Job drawing, mm, ordinate dimensions from the low corner. One solid piece. A direction names the side the tool comes from. Give positions to 0.01 mm unless a question says otherwise; leave off trailing zeros. Order: outer loops, then holes, each group sorted by start corner. A loop starts at its lowest first (then second) coordinate and runs counter-clockwise, first axis right, second up. Notation, with made-up numbers: M -37.5,24 L -3.5,24 A24 cw -3.5,47 Z; hole C 68.5,-38 d3. An arc over 180 degrees is marked long. Use CSV: the item, a comma, the result in double quotes. Start each with the question number.
Item 1: Band-saw the part on A-A on x = 38.5. Write the cut outline in (y, z) (3 decimals), plus the area to 3 significant figures.
Item 2: Band-saw the part on D-D on x = 7. Write the cut outline in (y, z) (3 decimals).
Item 3: Band-saw the part on B-B on y = 1.55. Write the cut outline in (x, z), plus the area to 3 significant figures.
Item 4: Which spindle directions (+Z, -Z, +X, -X, +Y, -Y) get a long thin tool onto all of the face, cutting with end or side? Do the marked faces 1, 2, 3 and 4. Say none if no direction does.
Item 5: Wall check: line 1 along Z through (x, y) = (34.5, 2.6); line 2 along X through (y, z) = (2, 51). Give the ranges that are in metal, low to high.
Item 6: Pin check, flat tips, straight feed: P1, Ø1, axis at x = 48.5, y = 2, coming from the -Z side (3 decimals); P2, Ø1, axis at x = 43.5, y = 2, coming from the +Z side (3 decimals); P3, Ø2, axis at y = 4, z = 14.5, coming from the -X side. Stop position of each tip, or through.
Item 7: Band-saw the part on C-C on z = 66.5. Write the cut outline in (x, y) (3 decimals).
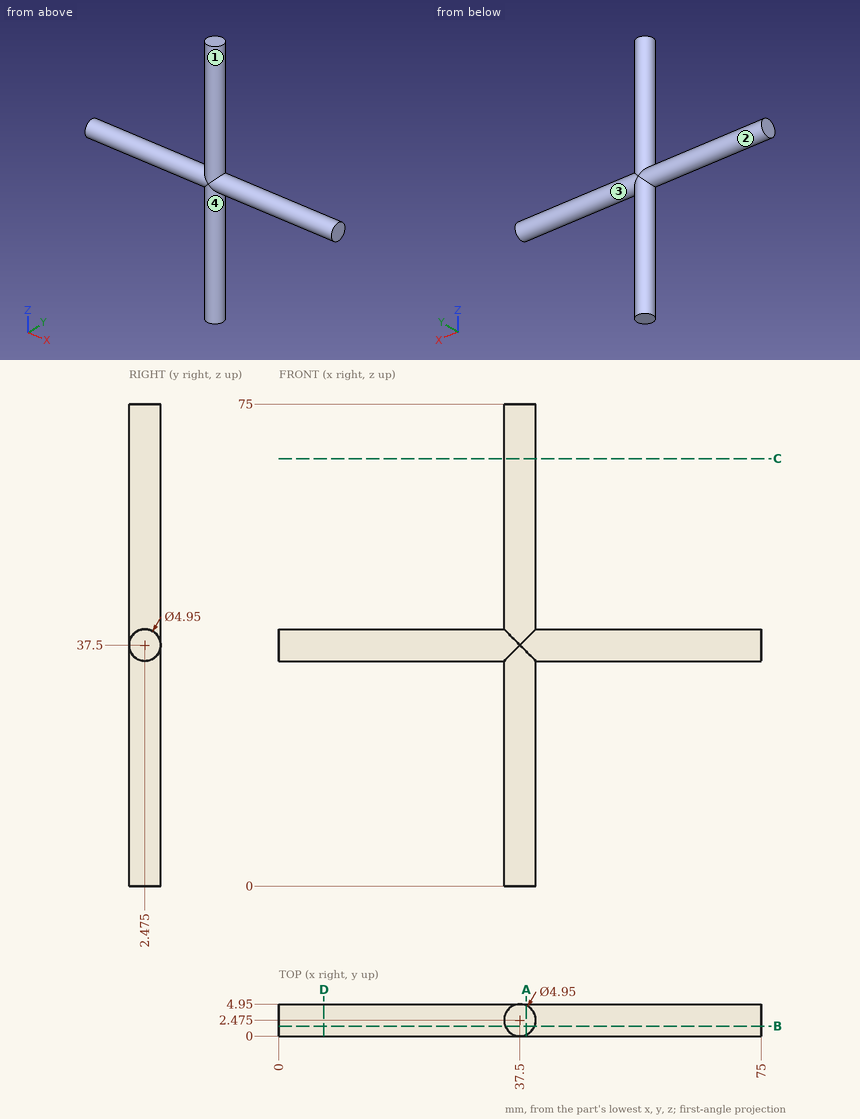
Model answer:
1,outline,"M 0.211,0 L 4.739,0 L 4.739,36.5 A2.475 ccw 4.739,38.5 L 4.739,75 L 0.211,75 L 0.211,38.5 A2.475 ccw 0.211,36.5 Z"
1,area,"340 mm^2"
2,outline,"C 2.475,37.5 d4.95"
3,outline,"M 0,35.2 L 35.2,35.2 L 35.2,0 L 39.8,0 L 39.8,35.2 L 75,35.2 L 75,39.8 L 39.8,39.8 L 39.8,75 L 35.2,75 L 35.2,39.8 L 0,39.8 Z"
3,area,"668 mm^2"
4,face 1,"+Z"
4,face 2,"-X"
4,face 3,"+X"
4,face 4,"-Z"
5,line 1,"z = 35.03 to 39.97"
5,line 2,"x = 35.07 to 39.93"
6,P1,"stops at z = 35.025"
6,P2,"stops at z = 39.975"
6,P3,"stops at x = 35.08"
7,outline,"C 37.5,2.475 d4.95"
